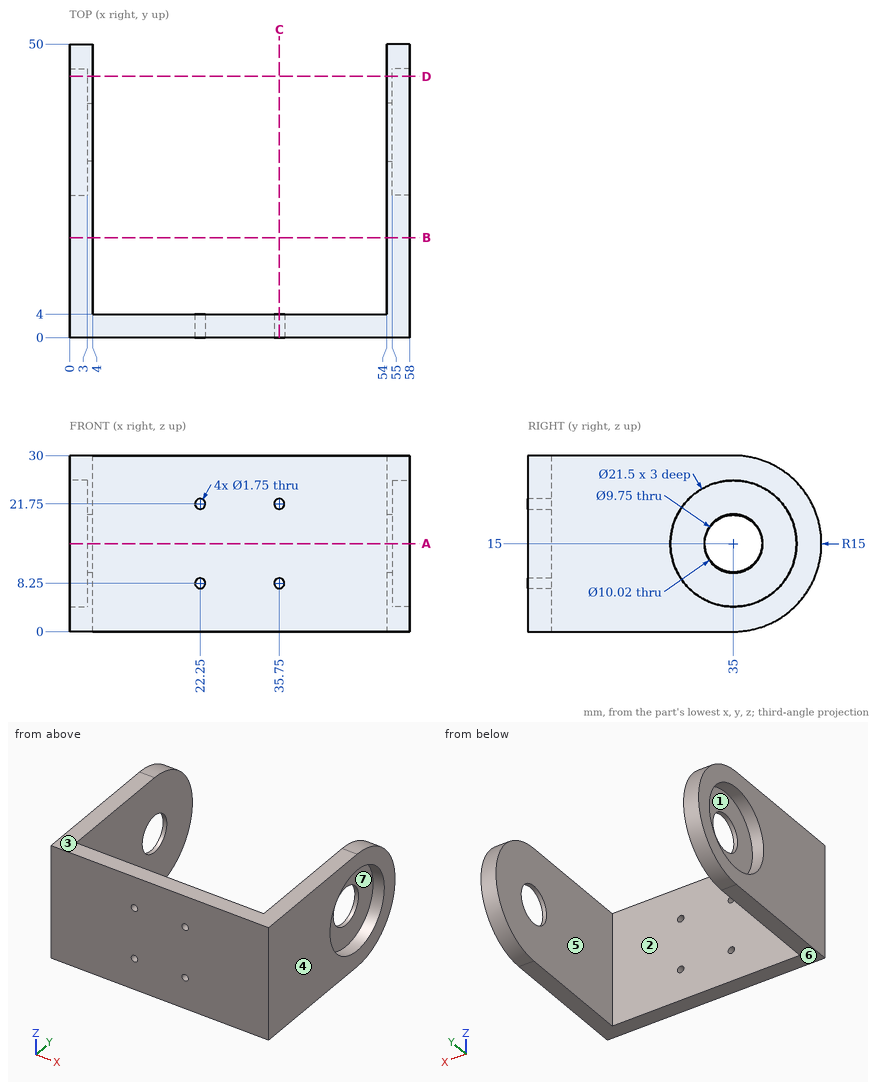
Input: dimensioned drawing with shaded views. Units: mm. Origin: part minimum x, y, z. A direction names the side the tool comes from. Give positions to 0.01 mm unless a question says otherwise; leave off trailing zeros. Order: outer loops, then holes, each group sorted by start corner. A loop starts at its lowest first (then second) coordinate and runs counter-clockwise, first axis right, second up. Notation, with made-up numbers: (5.25, 59) -> (54.25, 59) arc R21 cw to (54.25, 85) -> close; hole circle Ø10 at (82.5, -29.5). An arc over 180 degrees is marked (long way). Answer as a JSON object with one key per item and string values.
Q1. First-contact query: pin 1 (1.1 mm diameter, centred on x = 35.75, z = 21.75, fed in from +Y); pin 2 (6.5 mm diameter, centred on y = 33, z = 11, fed in from -X); pin 3 (1 mm diameter, centred on y = 29.5, z = 10.5, fed in from +X). Flat tips, straight axial feed; report the tip coordinate or a pass-through.
Entries:
{"pin 1": "passes through", "pin 2": "stops at x = 3", "pin 3": "stops at x = 55"}
Q2. Section A-A (z = 15). Output: boundary loops of the cut face in (x, y) (3 decimals), plus the area to 3 significant figures.
Entries:
{"outline": "(0, 0) -> (58, 0) -> (58, 24.25) -> (55, 24.25) -> (55, 29.99) -> (54, 29.99) -> (54, 4) -> (4, 4) -> (4, 30.125) -> (3, 30.125) -> (3, 24.25) -> (0, 24.25) -> close; (0, 45.75) -> (3, 45.75) -> (3, 39.875) -> (4, 39.875) -> (4, 50) -> (0, 50) -> close; (54, 40.01) -> (55, 40.01) -> (55, 45.75) -> (58, 45.75) -> (58, 50) -> (54, 50) -> close", "area": "451 mm^2"}
Q3. Access query for the marked faces 5, 6 and 7. Directions: +Z, -Z, +X, -X, +Y, -Y. A direction counts if a zero-diameter tool reaches every point of the face in a straight line with its end or side. Return the directions, or none.
Entries:
{"face 5": "+Z, -Z, +Y", "face 6": "-Z, +X, -X, +Y, -Y", "face 7": "+X"}
Q4. Draft query along X for the marked faces 1, 2, 3 and 4. Return one class per face: released by +X, released by -X, zero draft, split by the parting line, or undercut.
Entries:
{"face 1": "released by -X", "face 2": "undercut", "face 3": "zero draft", "face 4": "released by +X"}
Q5. Material intervals for probe 1 along X at (y, z) = (2.2, 21.75) (3 decimals); probe 2 along Y at (x, z) = (54.2, 15); probe 3 along X at (y, z) = (29.5, 15.25), sorted ascending.
Entries:
{"probe 1": "x = 0 to 21.375, 23.125 to 34.875, 36.625 to 58", "probe 2": "y = 0 to 29.99, 40.01 to 50", "probe 3": "x = 3 to 4, 54 to 55"}
Q6. Section C-C (x = 35.75). Output: boundary loops of the cut face in (y, z) (3 decimals), plus the area to 3 significant figures.
Entries:
{"outline": "(0, 0) -> (4, 0) -> (4, 7.375) -> (0, 7.375) -> close; (0, 9.125) -> (4, 9.125) -> (4, 20.875) -> (0, 20.875) -> close; (0, 22.625) -> (4, 22.625) -> (4, 30) -> (0, 30) -> close", "area": "106 mm^2"}
Q7. Section B-B (y = 17). Output: boundary loops of the cut face in (x, z).
Entries:
{"outline": "(0, 0) -> (4, 0) -> (4, 30) -> (0, 30) -> close; (54, 0) -> (58, 0) -> (58, 30) -> (54, 30) -> close"}
Q8. Section D-D (y = 44.5). Output: boundary loops of the cut face in (x, z).
Entries:
{"outline": "(0, 3.39) -> (4, 3.39) -> (4, 26.61) -> (0, 26.61) -> (0, 20.03) -> (3, 20.03) -> (3, 9.97) -> (0, 9.97) -> close; (54, 3.39) -> (58, 3.39) -> (58, 9.97) -> (55, 9.97) -> (55, 20.03) -> (58, 20.03) -> (58, 26.61) -> (54, 26.61) -> close"}
